Autodesk Inventor part; units mm, degrees
ref_plane "YZ Plane" through (0, 0, 0) normal (1, 0, 0) x (0, 1, 0)
ref_plane "XZ Plane" through (0, 0, 0) normal (0, 1, 0) x (-1, 0, 0)
ref_plane "XY Plane" through (0, 0, 0) normal (0, 0, 1) x (1, 0, 0)
sketch "Sketch1" plane through (0, 0, 0) normal (0, 0, 1) x (1, 0, 0)
  line L0 (-95, -19) -> (95, -19)
  line L1 (95, -19) -> (95, 19)
  line L2 (95, 19) -> (-95, 19)
  line L3 (-95, 19) -> (-95, -19)
  line L4 (-95, -19) -> (95, 19) construction
  line L5 (95, -19) -> (-95, 19) construction
  line L6 (-35, -11.92) -> (25, -11.92)
  line L7 (25, -11.92) -> (25, -15)
  line L8 (25, -15) -> (-35, -15)
  line L9 (-35, -15) -> (-35, -11.92)
  line L10 (-35, -11.92) -> (25, -15) construction
  line L11 (25, -11.92) -> (-35, -15) construction
  line L12 (62.5251, 6.067) -> (58.933, 2.4749)
  line L13 (58.933, 2.4749) -> (67.4749, -6.067)
  line L14 (67.4749, -6.067) -> (71.067, -2.4749)
  line L15 (71.067, -2.4749) -> (62.5251, 6.067)
  line L16 (67.4749, 6.067) -> (71.067, 2.4749)
  line L17 (71.067, 2.4749) -> (62.5251, -6.067)
  line L18 (62.5251, -6.067) -> (58.933, -2.4749)
  line L19 (58.933, -2.4749) -> (67.4749, 6.067)
  line L20 (60.7291, -4.2709) -> (69.2709, 4.2709)
  line L21 (60.7291, 4.2709) -> (69.2709, -4.2709)
  line L22 (0, 0) -> (95, 0)
  point P0 (-5, -13.46)
  point P1 (-5, -11.92)
  point P2 (65, 0)
  point P3 (68.5921, 0)
  point P4 (65, -3.5921)
  point P5 (61.4079, 0)
  point P6 (65, 3.5921)
  dimension "d0" = 38
  dimension "d1" = 190
  dimension "d2" = 3.08
  dimension "d3" = 60
  dimension "d4" = 100
  dimension "d5" = 4
  dimension "d6" = 45
  dimension "d7" = 5.08
  dimension "d8" = 12.08
  dimension "d9" = 30
extrude "Plate1" add sketch "Sketch1" along normal blind 3 contours L15 L14 L21 L17 | L17 L21 L22 | L22 L20 L15 | L15 L20 L16 L17 | L3 L2 L1 L0 | L20 L21 L19 L15 | L15 L19 L16 L20 | L21 L14 L13 L17 | L17 L13 L20 L21 | L22 L19 L21 | L20 L13 L22 | L19 L21 L12 L15 | L17 L18 L20 L13 | L20 L18 L19 L13 | L19 L13 L12 L21
extrude "Cut1" cut sketch "Sketch1" along normal through all contours L15 L14 L21 L17 | L17 L21 L22 | L22 L20 L15 | L15 L20 L16 L17 | L20 L21 L19 L15 | L15 L19 L16 L20 | L21 L14 L13 L17 | L17 L13 L20 L21 | L22 L19 L21 | L20 L13 L22 | L19 L21 L12 L15 | L17 L18 L20 L13 | L20 L18 L19 L13 | L19 L13 L12 L21
pattern_linear "Rectangular Pattern1" count 6 spacing 25 along (-1, 0, 0) of "Cut1"
equation "\"d11\" = Thickness"
equation "\"d10\" = Thickness"
equation "\"BendRadius\" = Thickness"
equation "\"BendReliefWidth\" = Thickness"
equation "\"BendReliefDepth\" = 0.5 * Thickness"
equation "\"CornerReliefSize\" = 4 * Thickness"
equation "\"MinimumRemnant\" = 2 * Thickness"
equation "\"TransitionRadius\" = BendRadius"
equation "\"JacobiRadiusSize\" = BendRadius"
equation "\"GapSize\" = Thickness"
properties part number "Extension.2"
Could you check a few things on this model? Use its own coordinates, in mm. A direction names the side the tool comes from. Round coordinates to 2 decimals unless told otherwise and drop trailing zeros. Order: outer loops, then holes, each group sorted by start corner. A loop starts at its lowest first (then second) coordinate and runs counter-clockwise, first axis right, second up. Notation, with made-up numbers: M 74,88.5 L 92,88.5 A5 ccw 92,92.5 Z; hole C 83,-37.5 d9. An arc over 180 degrees is marked long. One line per question, with ' | ' between items. Start each with the question number.
(1) Please list where these lines run through material, in increasing order: line 1 along Y through (x, z) = (-7.5, 0.45); line 2 along Y through (x, z) = (3, 1.3); line 3 along Y through (x, z) = (62.5, 0.85).
(2) For faces 4 (the face through (-95, 0, 1)), 5 (the face through (-55.754, 4.296, 1.479)), which set-ups out of +Z, -Z, +X, -X, +Y, -Y let a thin tool reach every point of the face, with its end or its side?
(3) For P1, Ø2, axis at x = -31, y = 4.5, coming from the +Z side, with a flat end and sliding along its axis, tell me the tip position at first contact or that it passes through.
(4) Thinking about a two-plate mould opening in Y: for faces 1 (the face through (-1, -19, 1)), 2 (the face through (-39.246, 4.296, 1.479)), 3 (the face through (95, 0, 1)), which applies, +Y half, -Y half, draft (parallel to the pull), parting line (faces both ways), or undercut?
(5) Suppose I cut it at B-B on z = 0.95. Count the separate pieces of the cut face and the enclosed holes in it, then the cut area to 3 significant figures.
(6) Suppose I cut it at A-A on x = 23. List the corners of the cut face in (y, z) for me, then the cut area to 3 significant figures.
Geometry results:
1) line 1: -19 to -15, -11.92 to -6.04, 6.04 to 19 | line 2: -19 to -15, -11.92 to 19 | line 3: -19 to -6.04, 6.04 to 19
2) face 4: +Z, -Z, -X, +Y, -Y | face 5: +Z, -Z
3) P1: z = 3
4) face 1: -Y half | face 2: undercut | face 3: draft
5) separate pieces: 1 | enclosed holes: 7 | area: 6,450 mm²
6) outline: M -19,0 L -15,0 L -15,3 L -19,3 Z; M -11.92,0 L 19,0 L 19,3 L -11.92,3 Z | area: 105 mm²
